```python
from build123d import *

# Parameters (mm, degrees)
F1_DEPTH    = 25.4
F2_W        = 105.8882400393
F2_H        = 70.1928213239
F3_DEPTH    = 55.88
F4_W        = 46.9851754606
F4_H        = 70.1928213239
F5_DEPTH    = 33.782
F6_R        = 23.301989304
F7_DEPTH    = 35.56
F8_T1_DEPTH = 210.348554518
F8_T3_DEPTH = 210.348554518
F9_R        = 19.8729907894
F10_DEPTH   = 207.5309093164


# Not quite as in the source:
# - a fillet or chamfer that OpenCascade refuses, or shapes differently, is made with other operations: its cross-section is extruded or revolved along the edge and cut away or added


with BuildPart() as f1:
    # F0 (on Top) → F1 (new body)
    with BuildSketch(Plane.XY):
        with BuildLine():
            Line((-99.153496325, -55.7124875486), (99.153496325, -55.7124875486))
            Line((99.153496325, -55.7124875486), (99.153496325, -55.4322929717))
            ThreePointArc((99.153496325, -55.4322929717), (43.7212033534, 0), (99.153496325, 55.4322929717))
            Line((99.153496325, 55.4322929717), (99.153496325, 55.7124875486))
            Line((99.153496325, 55.7124875486), (-99.153496325, 55.7124875486))
            Line((-99.153496325, 55.7124875486), (-99.153496325, 55.5695868493))
            ThreePointArc((-99.153496325, 55.5695868493), (-59.8598646362, 39.2936316888), (-43.5839094758, 0))
            ThreePointArc((-43.5839094758, 0), (-59.8598646362, -39.2936316888), (-99.153496325, -55.5695868493))
            Line((-99.153496325, -55.5695868493), (-99.153496325, -55.7124875486))
        make_face()
        with BuildLine():
            Line((99.153496325, -22.3866111857), (99.153496325, -55.4322929717))
            ThreePointArc((99.153496325, -55.4322929717), (138.350046582, -39.196550257), (154.5857892967, 0))
            ThreePointArc((154.5857892967, 0), (138.350046582, 39.196550257), (99.153496325, 55.4322929717))
            Line((99.153496325, 55.4322929717), (99.153496325, 22.3866111857))
            ThreePointArc((99.153496325, 22.3866111857), (114.9832209022, 15.8297245772), (121.5401075107, 0))
            ThreePointArc((121.5401075107, 0), (114.9832209022, -15.8297245772), (99.153496325, -22.3866111857))
        make_face()
        with BuildLine():
            ThreePointArc((-99.153496325, 55.5695868493), (-154.7230831743, 0), (-99.153496325, -55.5695868493))
            Line((-99.153496325, -55.5695868493), (-99.153496325, -23.1719717835))
            ThreePointArc((-99.153496325, -23.1719717835), (-122.3254681085, 0), (-99.153496325, 23.1719717835))
            Line((-99.153496325, 23.1719717835), (-99.153496325, 55.5695868493))
        make_face()
        with BuildLine():
            ThreePointArc((99.153496325, 55.4322929717), (43.7212033534, 0), (99.153496325, -55.4322929717))
            Line((99.153496325, -55.4322929717), (99.153496325, -22.3866111857))
            ThreePointArc((99.153496325, -22.3866111857), (76.7668851393, 0), (99.153496325, 22.3866111857))
            Line((99.153496325, 22.3866111857), (99.153496325, 55.4322929717))
        make_face()
        with BuildLine():
            Line((-99.153496325, -23.1719717835), (-99.153496325, -55.5695868493))
            ThreePointArc((-99.153496325, -55.5695868493), (-59.8598646362, -39.2936316888), (-43.5839094758, 0))
            ThreePointArc((-43.5839094758, 0), (-59.8598646362, 39.2936316888), (-99.153496325, 55.5695868493))
            Line((-99.153496325, 55.5695868493), (-99.153496325, 23.1719717835))
            ThreePointArc((-99.153496325, 23.1719717835), (-82.7684379434, 16.3850583816), (-75.9815245415, 0))
            ThreePointArc((-75.9815245415, 0), (-82.7684379434, -16.3850583816), (-99.153496325, -23.1719717835))
        make_face()
    extrude(amount=F1_DEPTH)

    # F2 (on face) → F3 (join)
    with BuildSketch(Plane.XY.offset(25.4)):
        Rectangle(F2_W, F2_H)
    extrude(amount=F3_DEPTH)

    # F4 (on face) → F5 (cut)
    with BuildSketch(Plane.XY.offset(81.28)):
        Rectangle(F4_W, F4_H)
    extrude(amount=-F5_DEPTH, mode=Mode.SUBTRACT)

    # F6
    f6_edges = [f1.edges().sort_by_distance(p)[0] for p in [
        (-23.492588, 0, 47.498),
        (23.492588, 0, 47.498),
    ]]
    fillet(f6_edges, radius=F6_R)

    # F7 (add): faces of the model
    f7_faces = [f1.faces().sort_by_distance(p)[0] for p in [
        (-38.218353875, 0, 81.28),
        (38.218353875, 0, 81.28),
    ]]
    extrude(f7_faces, amount=F7_DEPTH)

    # F8: fillet of radius 36.1794044457 on 4 edges, made by hand

    # F8_s2 → F8_t1 (cut)
    with BuildSketch(Plane.YZ.offset(-143.392631134)):
        with BuildLine():
            ThreePointArc((-35.0964106619, 80.6605955543), (-24.4997084391, 106.2432977771), (1.0829937838, 116.84))
            Line((1.0829937838, 116.84), (-35.0964106619, 116.84))
            Line((-35.0964106619, 116.84), (-35.0964106619, 80.6605955543))
        make_face()
        with BuildLine():
            ThreePointArc((35.0964106619, 80.6605955543), (24.4997084391, 106.2432977771), (-1.0829937838, 116.84))
            Line((-1.0829937838, 116.84), (35.0964106619, 116.84))
            Line((35.0964106619, 116.84), (35.0964106619, 80.6605955543))
        make_face()
    extrude(amount=F8_T1_DEPTH, mode=Mode.SUBTRACT)

    # F8_s4 → F8_t3 (cut)
    with BuildSketch(Plane.YZ.offset(-66.955923384)):
        with BuildLine():
            ThreePointArc((-35.0964106619, 80.6605955543), (-24.4997084391, 106.2432977771), (1.0829937838, 116.84))
            Line((1.0829937838, 116.84), (-35.0964106619, 116.84))
            Line((-35.0964106619, 116.84), (-35.0964106619, 80.6605955543))
        make_face()
        with BuildLine():
            ThreePointArc((35.0964106619, 80.6605955543), (24.4997084391, 106.2432977771), (-1.0829937838, 116.84))
            Line((-1.0829937838, 116.84), (35.0964106619, 116.84))
            Line((35.0964106619, 116.84), (35.0964106619, 80.6605955543))
        make_face()
    extrude(amount=F8_T3_DEPTH, mode=Mode.SUBTRACT)

    # F9 (on face) → F10 (cut, through all)
    with BuildSketch(Plane(origin=(-52.9441200197, 0, 0), x_dir=(0, -1, 0), z_dir=(-1, 0, 0))):
        with Locations((0, 80.6605955543)):
            Circle(F9_R)
    extrude(amount=-F10_DEPTH, mode=Mode.SUBTRACT)


solid = f1.part
```
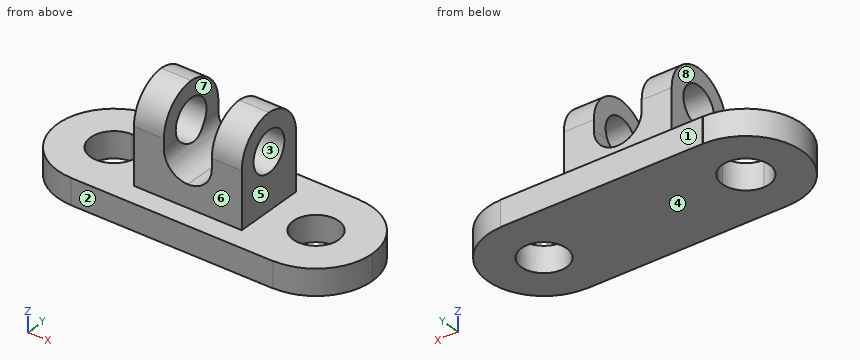
Part model, mm, in its own coordinate system. Face numbers are marked on the shaded views. A direction names the side the tool comes from. Round coordinates to 2 decimals unless told otherwise and drop trailing zeros. Loops run counter-clockwise (first coordinate to the right, second up) from the corner with the lowest first, then second, coordinate; pieces in that order, holes last. Notation, with made-up numbers: (31.25, 86) -> (43.25, 86) arc R27 cw to (43.25, 120) -> close; hole circle Ø2 at (6, -17.5). An arc over 180 degrees is marked (long way). Use CSV: the item, a comma, the result in double quotes. Start each with the question number.
1) Cut at B-B, the plane z = 110.5. Write the cut outline in (x, y).
2) Pull direction Y, two halves, no side cores. Call the marked faces 1, 2 and 3: +Y half, -Y half, draft (parallel to the pull), parting line (faces both ways), or undercut.
3) Wall check: L1, parallel to Z at x = 38.5, y = 0; L2, parallel to X at y = -15, z = 101; L3, parallel to X at y = 4, z = 15.5. Give the ranges that are in metal, low to high. Write a range as [from, to].
4) Cut at D-D, the plane x = -79. Write the cut outline in (y, z), plus the area to 3 significant figures.
5) Cut at C-C, the plane y = -10.5. Write the cut outline in (x, z), plus the area to 3 significant figures.
6) Cut at A-A, the plane x = -48. Write the cut outline in (y, z), plus the area to 3 significant figures.
7) Which spindle directions (+Z, -Z, +X, -X, +Y, -Y) get a long thin tool onto all of the face, cutting with end or side? Do the marked faces 4, 5, 6, 7 and 8. Say none if no direction does.
8) Drop flat-ended pins along their axis: P1, Ø10, axis at x = -55, y = 32.5, coming from the +Z side; P2, Ø3, axis at y = 37.5, z = 63.5, coming from the -X side; P3, Ø1, axis at y = -6.5, z = 18, coming from the -X side; P4, Ø3, axis at x = -38.5, y = 3, coming from the +Z side. Give the stop position or say it passes through.
Determined:
1,outline,"(-52.94, -19.38) -> (-23.49, -19.38) -> (-23.49, 19.38) -> (-52.94, 19.38) -> close; (23.49, -19.38) -> (52.94, -19.38) -> (52.94, 19.38) -> (23.49, 19.38) -> close"
2,face 1,"+Y half"
2,face 2,"-Y half"
2,face 3,"undercut"
3,L1,"z = [0, 60.79], [100.53, 116.82]"
3,L2,"x = [-52.94, -23.49], [23.49, 52.94]"
3,L3,"x = [-154.58, -121.98], [-76.33, 77.13], [121.18, 154.44]"
4,outline,"(-55.71, 0) -> (-11.44, 0) -> (-11.44, 25.4) -> (-55.71, 25.4) -> close; (11.44, 0) -> (55.71, 0) -> (55.71, 25.4) -> (11.44, 25.4) -> close"
4,area,"2,250 mm2"
5,outline,"(-153.72, 0) -> (-119.81, 0) -> (-119.81, 25.4) -> (-153.72, 25.4) -> close; (-78.5, 0) -> (79.38, 0) -> (79.38, 25.4) -> (52.94, 25.4) -> (52.94, 63.79) -> (22.41, 63.79) arc R23.3 cw to (0.19, 47.5) -> (-0.19, 47.5) arc R23.3 cw to (-22.41, 63.79) -> (-52.94, 63.79) -> (-52.94, 25.4) -> (-78.5, 25.4) -> close; (-52.94, 97.53) -> (-23.49, 97.53) -> (-23.49, 114.94) -> (-52.94, 114.94) -> close; (23.49, 97.53) -> (52.94, 97.53) -> (52.94, 114.94) -> (23.49, 114.94) -> close; (118.92, 0) -> (153.58, 0) -> (153.58, 25.4) -> (118.92, 25.4) -> close"
5,area,"10,300 mm2"
6,outline,"(-55.71, 0) -> (55.71, 0) -> (55.71, 25.4) -> (35.1, 25.4) -> (35.1, 80.66) arc R36.18 ccw to (0, 116.82) arc R36.18 ccw to (-35.1, 80.66) -> (-35.1, 25.4) -> (-55.71, 25.4) -> close; hole circle Ø39.75 at (0, 80.66)"
6,area,"7,450 mm2"
7,face 4,"-Z, +X, -X, +Y, -Y"
7,face 5,"+Z, +X, +Y, -Y"
7,face 6,"+Z, +X, -X, -Y"
7,face 7,"+Z, +Y, -Y"
7,face 8,"+Z, -X, +Y, -Y"
8,P1,"stops at z = 102.26"
8,P2,"passes through"
8,P3,"stops at x = -154.4"
8,P4,"stops at z = 116.75"
